Verification items for the finished model (mm, model axes). A direction names the side the tool comes from. Give positions to 0.01 mm unless a question says otherwise; leave off trailing zeros. Write each loop counter-clockwise with the first axis right and the second up, starting at its lowest first coordinate (ties: lowest second). Pieces come first, ordered by that corner, then holes. Notation, with made-up numbers: (-17, 78.25) -> (17, 78.25) arc R16 ccw to (17, 94.25) -> close; hole circle Ø11 at (-39.5, 20). An arc over 180 degrees is marked (long way). Use one line per item in the form item = value. Start each with the question number.
(1) Set-up check for faces 1 (the face through (49, 2, 2)), 2 (the face through (0, 46, 2)): record each of +Z, -Z, +X, -X, +Y, -Y from which the full face is reachable in a straight line by a thin tool's end or side.
(2) Section check C-C, the plane y = 84. Record the cut outline in (x, z), plus the area to 3 significant figures.
(3) Section check B-B, the plane z = 1.75. Record the cut outline in (x, y).
(4) Scan lines: L1, parallel to Y at x = 34.5, z = 2.8; L2, parallel to X at y = 38, z = 2.9. Record each from-to range of solid material in increasing order.
(5) Section check A-A, the plane x = 92.5. Record the cut outline in (y, z), plus the area to 3 significant figures.
(6) Release check for a two-part mould opening along Y. For faces 3 (the face through (49, 94, 2)), 4 (the face through (98, 46, 2)), 5 (the face through (1.6, 47.2, 0)) record: pulls with the +Y half, pulls with the -Y half, needs draft (parallel to the pull), parting line crosses it, or undercut.
from build123d import *

# Parameters (mm, degrees)
F0_W     = 100
F0_H     = 94
F1_DEPTH = 4
F2_T     = -2
F3_R     = 2


with BuildPart() as f1:
    # F0 (on Top) → F1 (new body)
    with BuildSketch(Plane.XY):
        with Locations((50, 47)):
            Rectangle(F0_W, F0_H)
    extrude(amount=F1_DEPTH)

    # F2
    f2_openings = [f1.faces().sort_by_distance(p)[0] for p in [
        (50, 47, 4),
        (50, 47, 0),
    ]]
    offset(amount=F2_T, openings=f2_openings)

    # F3
    f3_edges = [f1.edges().sort_by_distance(p)[0] for p in [
        (0, 94, 2),
        (0, 0, 2),
        (100, 94, 2),
        (100, 0, 2),
        (2, 92, 2),
        (2, 2, 2),
        (98, 92, 2),
        (98, 2, 2),
    ]]
    fillet(f3_edges, radius=F3_R)


solid = f1.part
Completed:
q1.face_1 = +Z, -Z
q1.face_2 = +Z, -Z, -X, +Y, -Y
q2.outline = (0, 0) -> (2, 0) -> (2, 4) -> (0, 4) -> close; (98, 0) -> (100, 0) -> (100, 4) -> (98, 4) -> close
q2.area = 16.0 mm²
q3.outline = (0, 2) arc R2 ccw to (2, 0) -> (98, 0) arc R2 ccw to (100, 2) -> (100, 92) arc R2 ccw to (98, 94) -> (2, 94) arc R2 ccw to (0, 92) -> close; hole (2, 4) arc R2 ccw to (4, 2) -> (96, 2) arc R2 ccw to (98, 4) -> (98, 90) arc R2 ccw to (96, 92) -> (4, 92) arc R2 ccw to (2, 90) -> close
q4.L1 = 0 to 2, 92 to 94
q4.L2 = 0 to 2, 98 to 100
q5.outline = (0, 0) -> (2, 0) -> (2, 4) -> (0, 4) -> close; (92, 0) -> (94, 0) -> (94, 4) -> (92, 4) -> close
q5.area = 16.0 mm²
q6.face_3 = pulls with the +Y half
q6.face_4 = undercut
q6.face_5 = needs draft
